```python
from build123d import *

# Parameters (mm, degrees)
BOSS_EXTRUDE1_DEPTH = 5
FILLET1_R           = 5
FILLET2_R           = 5
FILLET3_R           = 5
FILLET4_R           = 5
BOSS_EXTRUDE2_START = 70
BOSS_EXTRUDE2_DEPTH = 70
SKETCH3_W           = 49.2
SKETCH3_H           = 25
BOSS_EXTRUDE3_DEPTH = 55
SKETCH4_W           = 39.2
SKETCH4_H           = 50
CUT_EXTRUDE1_DEPTH  = 20


with BuildPart() as part:
    # Sketch1 → Boss-Extrude1 (new body)
    with BuildSketch(Plane.XY):
        Polygon((-30, 0), (30, 0), (80, -80), (80, -100), (-80, -100), (-80, -80), align=None)
    extrude(amount=BOSS_EXTRUDE1_DEPTH)

    # Fillet1
    fillet1_edges = [part.edges().sort_by_distance(p)[0] for p in [
        (-30, 0, 2.5),
    ]]
    fillet(fillet1_edges, radius=FILLET1_R)

    # Fillet2
    fillet2_edges = [part.edges().sort_by_distance(p)[0] for p in [
        (30, 0, 2.5),
    ]]
    fillet(fillet2_edges, radius=FILLET2_R)

    # Fillet3
    fillet3_edges = [part.edges().sort_by_distance(p)[0] for p in [
        (80, -80, 2.5),
    ]]
    fillet(fillet3_edges, radius=FILLET3_R)

    # Fillet4
    fillet4_edges = [part.edges().sort_by_distance(p)[0] for p in [
        (-80, -80, 2.5),
    ]]
    fillet(fillet4_edges, radius=FILLET4_R)

    # Sketch2 → Boss-Extrude2 (add)
    with BuildSketch(Plane.XY.offset(5).offset(BOSS_EXTRUDE2_START)):
        with BuildLine():
            Line((76, -100), (76, -81.433981132))
            ThreePointArc((76, -81.433981132), (75.961248746, -81.158298619), (75.847998304, -80.903982192))
            Line((75.847998304, -80.903982192), (28.076760096, -4.47000106))
            ThreePointArc((28.076760096, -4.47000106), (27.713530325, -4.125357519), (27.228761792, -4))
            Line((27.228761792, -4), (-27.228761792, -4))
            ThreePointArc((-27.228761792, -4), (-27.713530325, -4.125357519), (-28.076760096, -4.47000106))
            Line((-28.076760096, -4.47000106), (-75.847998304, -80.903982192))
            ThreePointArc((-75.847998304, -80.903982192), (-75.961248746, -81.158298619), (-76, -81.433981132))
            Line((-76, -81.433981132), (-76, -100))
            Line((-76, -100), (-80, -100))
            Line((-80, -100), (-80, -81.433981132))
            ThreePointArc((-80, -81.433981132), (-79.806243731, -80.055568567), (-79.23999152, -78.783986432))
            Line((-79.23999152, -78.783986432), (-31.468753312, -2.3500053))
            ThreePointArc((-31.468753312, -2.3500053), (-29.652604454, -0.626787594), (-27.228761792, 0))
            Line((-27.228761792, 0), (27.228761792, 0))
            ThreePointArc((27.228761792, 0), (29.652604454, -0.626787594), (31.468753312, -2.3500053))
            Line((31.468753312, -2.3500053), (79.23999152, -78.783986432))
            ThreePointArc((79.23999152, -78.783986432), (79.806243731, -80.055568567), (80, -81.433981132))
            Line((80, -81.433981132), (80, -100))
            Line((80, -100), (76, -100))
        make_face()
    extrude(amount=-BOSS_EXTRUDE2_DEPTH)

    # Sketch3 → Boss-Extrude3 (add)
    with BuildSketch(Plane(origin=(0, 0, 0), x_dir=(-1, 0, 0), z_dir=(0, 0, -1))):
        with Locations((0, -12.5)):
            Rectangle(SKETCH3_W, SKETCH3_H)
    extrude(amount=-BOSS_EXTRUDE3_DEPTH)

    # Sketch4 → Cut-Extrude1 (cut)
    with BuildSketch(Plane(origin=(0, 0, 0), x_dir=(1, 0, 0), z_dir=(0, 1, 0))):
        with Locations((0, -25)):
            Rectangle(SKETCH4_W, SKETCH4_H)
    extrude(amount=-CUT_EXTRUDE1_DEPTH, mode=Mode.SUBTRACT)


solid = part.part
```
Could you check a few things on this model? Use its own coordinates, in mm. A direction names the side the tool comes from. Round coordinates to 2 decimals unless told otherwise and drop trailing zeros. Loops run counter-clockwise (first coordinate to the right, second up) from the corner with the lowest first, then second, coordinate; pieces in that order, holes last. Notation, with made-up numbers: (19.5, -16) -> (28.5, -16) arc R19 cw to (28.5, 6) -> close; hole circle Ø6 at (78, 71). An arc over 180 degrees is marked (long way). One line per question, with ' | ' between items.
(1) If we section it at C-C on y = -58.5: List the corners of the cut face in (x, z) for me.
Model answer:
outline: (-66.56, 0) -> (66.56, 0) -> (66.56, 75) -> (61.85, 75) -> (61.85, 5) -> (-61.85, 5) -> (-61.85, 75) -> (-66.56, 75) -> close
(2) If we section it at A-A on z = 16: List the corners of the cut face in (x, y) for me, and give its area (3 significant figures).
Model answer:
outline: (-80, -100) -> (-76, -100) -> (-76, -81.43) arc R1 cw to (-75.85, -80.9) -> (-28.08, -4.47) arc R1 cw to (-27.23, -4) -> (-24.6, -4) -> (-24.6, -25) -> (24.6, -25) -> (24.6, -4) -> (27.23, -4) arc R1 cw to (28.08, -4.47) -> (75.85, -80.9) arc R1 cw to (76, -81.43) -> (76, -100) -> (80, -100) -> (80, -81.43) arc R5 ccw to (79.24, -78.78) -> (31.47, -2.35) arc R5 ccw to (27.23, 0) -> (19.6, 0) -> (19.6, -20) -> (-19.6, -20) -> (-19.6, 0) -> (-27.23, 0) arc R5 ccw to (-31.47, -2.35) -> (-79.24, -78.78) arc R5 ccw to (-80, -81.43) -> close | area: 1,370 mm^2
(3) If we section it at B-B on x = -62: List the corners of the cut face in (y, z) for me, and give its area (3 significant figures).
Model answer:
outline: (-100, 0) -> (-51.2, 0) -> (-51.2, 75) -> (-58.75, 75) -> (-58.75, 5) -> (-100, 5) -> close | area: 772 mm^2
(4) If I drill on probe 1 along X at (y, z) = (-9, 40) (3 decimals); probe 2 along X at (y, z) = (-4.5, 45.5); probe 3 along Z at (x, y) = (-48, -60.5), over which ranges is the centre line in solid material (lowest first)?
Model answer:
probe 1: x = -35.625 to -30.908, -24.6 to -19.6, 19.6 to 24.6, 30.908 to 35.625 | probe 2: x = -32.81 to -28.1, -24.6 to -19.6, 19.6 to 24.6, 28.1 to 32.81 | probe 3: z = 0 to 5
(5) For pin 1 Ø4 at (x, z) = (-5, 23.5) entering from +Y; pin 2 Ø4 at (x, z) = (-18.5, 55.5) entering from -Y; pin 3 Ø10.5 at (x, y) = (-3, -11) entering from +Z, each with a flat end and sliding along its axis, tell me the tip position at first contact or that it passes through.
Model answer:
pin 1: stops at y = -20 | pin 2: stops at y = -25 | pin 3: stops at z = 55
(6) If we section it at D-D on z = 59.5: List the corners of the cut face in (x, y) for me.
Model answer:
outline: (-80, -100) -> (-76, -100) -> (-76, -81.43) arc R1 cw to (-75.85, -80.9) -> (-28.08, -4.47) arc R1 cw to (-27.23, -4) -> (27.23, -4) arc R1 cw to (28.08, -4.47) -> (75.85, -80.9) arc R1 cw to (76, -81.43) -> (76, -100) -> (80, -100) -> (80, -81.43) arc R5 ccw to (79.24, -78.78) -> (31.47, -2.35) arc R5 ccw to (27.23, 0) -> (-27.23, 0) arc R5 ccw to (-31.47, -2.35) -> (-79.24, -78.78) arc R5 ccw to (-80, -81.43) -> close
(7) For faces 1 (the face through (-76, -91, 40)), 2 (the face through (-19.6, -10, 25)), 3 (the face through (0, -2, 75)), which set-ups out of +Z, -Z, +X, -X, +Y, -Y let a thin tool reach every point of the face, with its end or its side?
Model answer:
face 1: +Z, -Y | face 2: -Z, +Y | face 3: +Z, +X, -X, +Y, -Y
